```python
from build123d import *

# Parameters (mm, degrees)
SKETCH2_W                          = 63.5
SKETCH2_H                          = 31.75
BOSS_EXTRUDE1_DEPTH                = 31.75
F_29_32_0_90625_DIAMETER_HOLE1_D   = 23.01875
BOSS_EXTRUDE2_DEPTH                = 5.08
F_7_16_0_4375_DIAMETER_HOLE1_D     = 11.1125
F_7_16_0_4375_DIAMETER_HOLE1_DEPTH = 25.4
F_7_16_0_4375_DIAMETER_HOLE1_TIP   = 3.338531814


with BuildPart() as part:
    # Sketch2 → Boss-Extrude1 (new body)
    with BuildSketch(Plane(origin=(0, 0, 0), x_dir=(1, 0, 0), z_dir=(0, 1, 0))):
        Rectangle(SKETCH2_W, SKETCH2_H)
    extrude(amount=BOSS_EXTRUDE1_DEPTH)

    # 29/32 (0.90625) Diameter Hole1 (through all)
    with Locations(Plane(origin=(31.75, 0, 0), x_dir=(0, 0, -1), z_dir=(1, 0, 0))):
        with Locations((0, 15.875)):
            Hole(F_29_32_0_90625_DIAMETER_HOLE1_D / 2)

    # Sketch10 → Boss-Extrude2 (add)
    with BuildSketch(Plane.XY.offset(15.875)):
        Polygon((9.525, 11.1125), (-9.525, 20.6375), (-9.525, 6.35), (9.525, 6.35), align=None)
        Polygon((-9.525, 25.4), (-9.525, 20.6375), (9.525, 11.1125), (9.525, 25.4), align=None)
    extrude(amount=BOSS_EXTRUDE2_DEPTH)

    # 7/16 (0.4375) Diameter Hole1
    with Locations(Plane.XY.offset(20.955)):
        with Locations((0, 15.875)):
            Hole(F_7_16_0_4375_DIAMETER_HOLE1_D / 2, depth=F_7_16_0_4375_DIAMETER_HOLE1_DEPTH)
            with Locations((0, 0, -(F_7_16_0_4375_DIAMETER_HOLE1_DEPTH + F_7_16_0_4375_DIAMETER_HOLE1_TIP / 2))):  # 118° drill point
                Cone(0, F_7_16_0_4375_DIAMETER_HOLE1_D / 2, F_7_16_0_4375_DIAMETER_HOLE1_TIP, mode=Mode.SUBTRACT)


solid = part.part
```
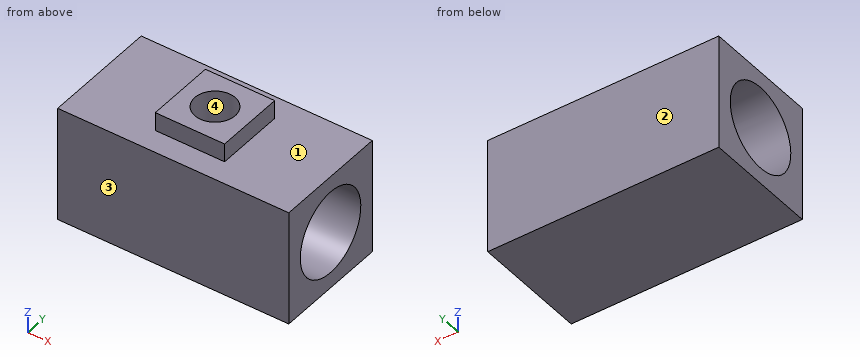
Could you check a few things on this model? Use its own coordinates, in mm. Face numbers are marked on the shaded views. Coordinates: 2 decimals unless noted, no trailing zeros. Order: outer loops, then holes, each group sorted by start corner. A loop starts at its lowest first (then second) coordinate and runs counter-clockwise, first axis right, second up. Notation, with made-up numbers: M 75,6.5 L 134,6.5 A32 cw 134,40.5 Z; hole C 11.5,-29 d2. An arc over 180 degrees is marked long. Use a Markdown table: item, result. Add a question column.
Q1. I'm going to push flat-ended pins straight in: pin 1 (1.5 mm diameter, centred on y = 12, z = 18, fed in from -X) (3 decimals); pin 2 (10 mm diameter, centred on x = 20.5, y = 14, fed in from +Z) (3 decimals); pin 3 (1.5 mm diameter, centred on y = 15.5, z = 19, fed in from +X) (3 decimals). Where does each tip first touch, or does it pass through?
Q2. We'd pull the mould along Y, two halves only. Please class the marked faces 1, 2, 3 and 4: pulls with the +Y half, pulls with the -Y half, needs draft (parallel to the pull), parting line crosses it, or undercut.
Q3. I want a section at D-D on y = 9.5. List the corners of the cut face in (x, z) for me (3 decimals), then the cut area to 3 significant figures.
Q4. If I drill on L1, parallel to Y at x = -14.5, z = 0; L2, parallel to X at y = 21.5, z = 17 (3 decimals); L3, parallel to Z at x = 27, y = 21 (3 decimals), over which ranges is the centre line in solid material (lowest first)?
Q5. I want a section at B-B on x = -7. List the corners of the cut face in (y, z) for me (3 decimals), then the cut area to 3 significant figures.
Q6. I want a section at A-A on z = 0. List the corners of the cut face in (x, y) for me, then the cut area to 3 significant figures.
Checked values:
| question | item | result |
|---|---|---|
| 1 | pin 1 | x = -9.525 |
| 1 | pin 2 | z = 15.875 |
| 1 | pin 3 | x = 9.525 |
| 2 | face 1 | needs draft |
| 2 | face 2 | pulls with the +Y half |
| 2 | face 3 | pulls with the -Y half |
| 2 | face 4 | undercut |
| 3 | outline | M -31.75,-15.875 L 31.75,-15.875 L 31.75,-9.583 L -31.75,-9.583 Z; M -31.75,9.583 L 31.75,9.583 L 31.75,15.875 L 9.525,15.875 L 9.525,20.955 L -9.525,20.955 L -9.525,15.875 L -31.75,15.875 Z |
| 3 | area | 896 mm² |
| 4 | L1 | 0 to 4.37, 27.38 to 31.75 |
| 4 | L2 | -9.525 to 9.525 |
| 4 | L3 | -15.875 to -10.305, 10.305 to 15.875 |
| 5 | outline | M 0,-15.875 L 31.75,-15.875 L 31.75,15.875 L 25.4,15.875 L 25.4,20.955 L 6.35,20.955 L 6.35,15.875 L 0,15.875 Z; hole C 15.875,0 d23.019 |
| 5 | area | 689 mm² |
| 6 | outline | M -31.75,0 L 31.75,0 L 31.75,4.37 L -31.75,4.37 Z; M -31.75,27.38 L 31.75,27.38 L 31.75,31.75 L -31.75,31.75 Z |
| 6 | area | 554 mm² |
